Geometry: final body of the model. Coordinates: model frame, mm. A direction names the side the tool comes from. Give positions to 0.01 mm unless a question says otherwise; leave off trailing zeros. Write each loop counter-clockwise with the first axis right and the second up, starting at its lowest first coordinate (ties: lowest second). Pieces come first, ordered by that corner, then holes. Notation, with made-up numbers: (54.25, -4) -> (93.25, -4) arc R4 ccw to (93.25, 0) -> close; hole circle Ø2 at (1, 89). An arc over 180 degrees is marked (long way). Answer in a Markdown table with one row per item. Add a question column.
Item 1: Access query for faces 1 (the flat face through (-8, -15.995, 17)), 2 (the flat face through (5, -28.735, 17)). Directions: +Z, -Z, +X, -X, +Y, -Y. A direction counts if a zero-diameter tool reaches every point of the face in a straight line with its end or side. Return the directions, or none.
Item 2: Draft query along X for faces 3 (the flat face through (-15.929, 22, 17)), 4 (the flat face through (19, -6, 22.22)), 5 (the cylindrical face through (-0.73, -24.27, 16.74)). Return one class per face: +X half, -X half, draft (parallel to the pull), parting line (faces both ways), or undercut.
Item 3: Section query A-A on x = 3.5. Output: boundary loops of the cut face in (y, z) (3 decimals).
Item 4: Material intervals for probe 1 along Y at (x, z) = (-7, 12) (3 decimals); probe 2 along Y at (x, z) = (0.5, 19.75) (3 decimals); probe 3 along Y at (x, z) = (-1.5, 17) (3 decimals), sorted ascending. Write a range as from..to.
Item 5: Section query D-D on y = -10. Output: boundary loops of the cut face in (x, z).
Item 6: Section query B-B on z = 16.25. Output: boundary loops of the cut face in (x, y) (3 decimals), plus the area to 3 significant figures.
Item 7: Section query C-C on y = -1. Output: boundary loops of the cut face in (x, z), plus the area to 3 significant figures.
Item 8: First-contact query: P1, Ø1, axis at y = -3.5, z = 13, coming from the -X side; P2, Ø7, axis at x = -0.13, y = 21.32, coming from the +Z side. Flat tips, straight axial feed; report the tip coordinate or a pass-through.
```python
from build123d import *

# Parameters (mm, degrees)
ESBO_O1_W                = 53.82
ESBO_O1_H                = 57.47
RESSALTO_EXTRUS_O1_DEPTH = 11.11
RESSALTO_EXTRUS_O2_DEPTH = 11.11
ESBO_O4_R                = 2.755
CORTE_EXTRUS_O2_DEPTH    = 11.11
ESBO_O3_W                = 53.82
ESBO_O3_H                = 57.47
CORTE_EXTRUS_O3_DEPTH    = 11.11
ESBO_O5_W                = 42.839074837
ESBO_O5_H                = 1
CORTE_EXTRUS_O4_DEPTH    = 11.11


with BuildPart() as part:
    # Esboço1 → Ressalto-extrusão1 (new body)
    with BuildSketch(Plane.XY):
        Rectangle(ESBO_O1_W, ESBO_O1_H)
    extrude(amount=RESSALTO_EXTRUS_O1_DEPTH)

    # Esboço2 → Ressalto-extrusão2 (add)
    with BuildSketch(Plane.XY.offset(11.11)):
        with BuildLine():
            Line((0.065925163, -15.995), (-15.929074837, -15.995))
            Line((-15.929074837, -15.995), (-15.929074837, -28.735))
            Line((-15.929074837, -28.735), (0, -28.735))
            Line((0, -28.735), (26.91, -28.735))
            Line((26.91, -28.735), (26.91, 28.735))
            Line((26.91, 28.735), (0, 28.735))
            Line((0, 28.735), (-15.929074837, 28.735))
            Line((-15.929074837, 28.735), (-15.929074837, 15.995))
            Line((-15.929074837, 15.995), (0.065925163, 15.995))
            ThreePointArc((0.065925163, 15.995), (16.060925163, 0), (0.065925163, -15.995))
        make_face()
    extrude(amount=RESSALTO_EXTRUS_O2_DEPTH)

    # Esboço4 → Corte-extrusão2 (cut)
    with BuildSketch(Plane.XY.offset(22.22)):
        with Locations((21.318136928, -0.131850449)):
            Circle(ESBO_O4_R)
        with Locations((-0.131863072, -21.581850449)):
            Circle(ESBO_O4_R)
        with Locations((-0.131863072, 21.318149551)):
            Circle(ESBO_O4_R)
    extrude(amount=-CORTE_EXTRUS_O2_DEPTH, mode=Mode.SUBTRACT)

    # Esboço3 → Corte-extrusão3 (cut)
    with BuildSketch(Plane(origin=(0, 0, 0), x_dir=(-1, 0, 0), z_dir=(0, 0, -1))):
        Rectangle(ESBO_O3_W, ESBO_O3_H)
    extrude(amount=-CORTE_EXTRUS_O3_DEPTH, mode=Mode.SUBTRACT)

    # Esboço5 → Corte-extrusão4 (cut)
    with BuildSketch(Plane(origin=(0, 0, 11.11), x_dir=(-1, 0, 0), z_dir=(0, 0, -1))):
        with Locations((-5.490462581, 28.235)):
            Rectangle(ESBO_O5_W, ESBO_O5_H)
    extrude(amount=-CORTE_EXTRUS_O4_DEPTH, mode=Mode.SUBTRACT)


solid = part.part
```
Findings below:
| question | item | result |
|---|---|---|
| 1 | face 1 | +Z, -Z, -X |
| 1 | face 2 | +Z, -Z, +X, -X, -Y |
| 2 | face 3 | -X half |
| 2 | face 4 | draft |
| 2 | face 5 | undercut |
| 3 | outline | (-28.735, 11.11) -> (-15.622, 11.11) -> (-15.622, 22.22) -> (-28.735, 22.22) -> close; (15.622, 11.11) -> (27.735, 11.11) -> (27.735, 22.22) -> (15.622, 22.22) -> close |
| 4 | probe 1 | y = -28.735..-15.995, 15.995..27.735 |
| 4 | probe 2 | y = -28.735..-24.263, -18.9..-15.989, 15.989..18.637, 24..27.735 |
| 4 | probe 3 | y = -28.735..-23.973, -19.191..-15.995, 15.995..18.927, 23.709..27.735 |
| 5 | outline | (12.55, 11.11) -> (26.91, 11.11) -> (26.91, 22.22) -> (12.55, 22.22) -> close |
| 6 | outline | (-15.929, -28.735) -> (26.91, -28.735) -> (26.91, 27.735) -> (-15.929, 27.735) -> (-15.929, 15.995) -> (0.066, 15.995) arc R15.995 cw to (0.066, -15.995) -> (-15.929, -15.995) -> close; hole circle Ø5.51 at (-0.132, -21.582); hole circle Ø5.51 at (-0.132, 21.318); hole circle Ø5.51 at (21.318, -0.132) |
| 6 | area | 1,430 mm^2 |
| 7 | outline | (16.03, 11.11) -> (18.7, 11.11) -> (18.7, 22.22) -> (16.03, 22.22) -> close; (23.93, 11.11) -> (26.91, 11.11) -> (26.91, 22.22) -> (23.93, 22.22) -> close |
| 7 | area | 62.8 mm^2 |
| 8 | P1 | stops at x = 15.55 |
| 8 | P2 | stops at z = 22.22 |
